from build123d import *

# Parameters (mm, degrees)
PAD_DEPTH       = 45
SKETCH001_R     = 1
POCKET_DEPTH    = 5
SKETCH002_R     = 0.825
POCKET001_DEPTH = 10
SKETCH004_R     = 1.5
POCKET003_DEPTH = 5
SKETCH005_W     = 50
SKETCH005_H     = 25
POCKET004_DEPTH = 5
SKETCH006_R     = 2
POCKET005_DEPTH = 2
SKETCH007_R     = 3
POCKET006_DEPTH = 3


with BuildPart() as part:
    # Sketch → Pad (new body)
    with BuildSketch(Plane.YZ):
        Polygon((0, 0), (0, 83), (24, 83), (24, 53), (27, 53), (27, 86), (0, 86), (0, 136), (-5, 136), (-5, 0), align=None)
    extrude(amount=PAD_DEPTH)

    # Sketch001 (on Face1 of Pad) → Pocket (cut)
    with BuildSketch(Plane(origin=(0, -5, 0), x_dir=(0, 0, -1), z_dir=(0, -1, 0))):
        with Locations((-57, 42.5)):
            Circle(SKETCH001_R)
        with Locations((-39, 42.5)):
            Circle(SKETCH001_R)
        with Locations((-57, 2.5)):
            Circle(SKETCH001_R)
        with Locations((-39, 2.5)):
            Circle(SKETCH001_R)
    extrude(amount=-POCKET_DEPTH, mode=Mode.SUBTRACT)

    # Sketch002 (on Face5 of Pocket) → Pocket001 (cut)
    with BuildSketch(Plane.YX):
        with Locations((-2.5, 35)):
            Circle(SKETCH002_R)
        with Locations((-2.5, 10)):
            Circle(SKETCH002_R)
    extrude(amount=-POCKET001_DEPTH, mode=Mode.SUBTRACT)

    # Sketch004 → Pocket003 (cut)
    with BuildSketch(Plane(origin=(0, -5, 0), x_dir=(0, 0, -1), z_dir=(0, -1, 0))):
        with Locations((-126, 35)):
            Circle(SKETCH004_R)
        with Locations((-106, 35)):
            Circle(SKETCH004_R)
    extrude(amount=-POCKET003_DEPTH, mode=Mode.SUBTRACT)

    # Sketch005 (on Face1 of Pocket003) → Pocket004 (cut)
    with BuildSketch(Plane(origin=(0, -5, 0), x_dir=(0, 0, -1), z_dir=(0, -1, 0))):
        with Locations((-111, 12.5)):
            Rectangle(SKETCH005_W, SKETCH005_H)
    extrude(amount=-POCKET004_DEPTH, mode=Mode.SUBTRACT)

    # Sketch006 (on Face20 of Pocket004) → Pocket005 (cut)
    with BuildSketch(Plane.ZX):
        with Locations((39, 42.5)):
            Circle(SKETCH006_R)
        with Locations((57, 42.5)):
            Circle(SKETCH006_R)
        with Locations((39, 2.5)):
            Circle(SKETCH006_R)
        with Locations((57, 2.5)):
            Circle(SKETCH006_R)
    extrude(amount=-POCKET005_DEPTH, mode=Mode.SUBTRACT)

    # Sketch007 (on Face14 of Pocket005) → Pocket006 (cut)
    with BuildSketch(Plane.ZX):
        with Locations((106, 35)):
            Circle(SKETCH007_R)
        with Locations((126, 35)):
            Circle(SKETCH007_R)
    extrude(amount=-POCKET006_DEPTH, mode=Mode.SUBTRACT)


solid = part.part
Read the model definition and answer for the solid it produces. Units are mm, in the model's axes. A direction names the side the tool comes from. Give positions to 0.01 mm unless a question says otherwise; leave off trailing zeros. Write each loop counter-clockwise with the first axis right and the second up, starting at its lowest first coordinate (ties: lowest second). Pieces come first, ordered by that corner, then holes. Notation, with made-up numbers: (67.25, 59.25) - (89.25, 59.25) arc R31 ccw to (89.25, 86.25) - close; hole circle Ø11 at (51.5, 16). An arc over 180 degrees is marked (long way). Use CSV: the item, a comma, the result in double quotes. Start each with the question number.
(1) Find section D-D (z = 26). Give the vertices of the cut face in (x, y).
(2) Determine the mould class of faces 4 (the flat face through (0, -1, 50)), 5 (the flat face through (35, -2, 136)), 6 (the flat face through (33.7, -3, 107.3)) for opening direction X: +X half, -X half, draft (parallel to the pull), parting line (faces both ways), or undercut.
(3) Find section B-B (x = 13.5). Give the vertices of the cut face in (y, z), plus the area to 3 significant figures.
(4) Find section A-A (z = 106). Give the vertices of the cut face in (x, y), plus the area to 3 significant figures.
(5) Given P1, Ø5, axis at x = 33, y = 8, coming from the -Z side; P2, Ø5.5, axis at y = -3.5, z = 120, coming from the -X side; P3, Ø8, axis at x = 35, z = 126, coming from the +Y side; P4, Ø1.2, axis at x = 42.5, z = 39, coming from the +Y side, each flat-ended and moving along its own axis, determine where each tip first touches the part or whether it passes through.
(6) Consider line 1 along X through (y, z) = (-0.35, 57); line 2 along X through (y, z) = (-2.8, 57); line 3 along Y through (x, z) = (6.5, 62). Determine where each line is inside the solid, lowest interval first.
(7) For faces 1 (the cylindrical face through (40.548, -0.986, 38.566)), 2 (the flat face through (35, 0, 111)), 3 (the flat face through (22, 0, 41)), determine the directions among +Z, -Z, +X, -X, +Y, -Y from which every point of the face is accessible in a straight line to the end or side of a thin tool.
(8) Find section C-C (y = 9). Give the vertices of the cut face in (x, z).
Findings below:
1,outline,"(0, -5) - (45, -5) - (45, 0) - (0, 0) - close"
2,face 4,"-X half"
2,face 5,"draft"
2,face 6,"undercut"
3,outline,"(-5, 0) - (0, 0) - (0, 83) - (24, 83) - (24, 53) - (27, 53) - (27, 86) - (-5, 86) - close"
3,area,"601 mm2"
4,outline,"(25, -5) - (33.5, -5) - (33.5, -3) - (32, -3) - (32, 0) - (25, 0) - close; (36.5, -5) - (45, -5) - (45, 0) - (38, 0) - (38, -3) - (36.5, -3) - close"
4,area,"76.0 mm2"
5,P1,"z = 83"
5,P2,"x = 25"
5,P3,"y = 0"
5,P4,"through"
6,line 1,"0 to 0.5, 4.5 to 40.5, 44.5 to 45"
6,line 2,"0 to 1.5, 3.5 to 41.5, 43.5 to 45"
6,line 3,"-5 to 0, 24 to 27"
7,face 1,"+Y"
7,face 2,"+Z, +X, -X, +Y"
7,face 3,"-Z, +X, -X"
8,outline,"(0, 83) - (45, 83) - (45, 86) - (0, 86) - close"
